Design review of the part built by this model. Coordinates are the model's own, in mm. Face numbers are marked on the shaded views. Round coordinates to 2 decimals unless told otherwise and drop trailing zeros. Order: outer loops, then holes, each group sorted by start corner. A loop starts at its lowest first (then second) coordinate and runs counter-clockwise, first axis right, second up.
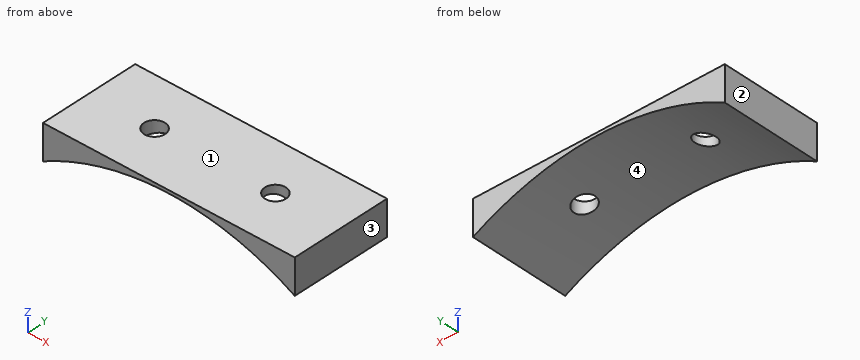
from build123d import *

# Parameters (mm, degrees)
EXTRUDE_1_DEPTH     = 20
SKETCH_2_R          = 2.1
CUT_EXTRUDE_1_DEPTH = 20


with BuildPart() as part:
    # Эскиз1 → Бобышка-Вытянуть1 (new body)
    with BuildSketch(Plane(origin=(0, 0, 0), x_dir=(1, 0, 0), z_dir=(0, 1, 0))):
        with BuildLine():
            Line((-25, -46.165463282), (-25, -53.1))
            Line((-25, -53.1), (25, -53.1))
            Line((25, -53.1), (25, -46.165463282))
            ThreePointArc((25, -46.165463282), (0, -52.5), (-25, -46.165463282))
        make_face()
    extrude(amount=EXTRUDE_1_DEPTH)

    # Эскиз2 → Вырез-Вытянуть1 (cut)
    with BuildSketch(Plane.XY.offset(53.1)):
        with Locations((-12, 10)):
            Circle(SKETCH_2_R)
        with Locations((12, 10)):
            Circle(SKETCH_2_R)
    extrude(amount=-CUT_EXTRUDE_1_DEPTH, mode=Mode.SUBTRACT)


solid = part.part
1) The part is to be moulded in two halves that separate along X. For the marked faces 1, 2, 3 and 4, say which applies: released by +X, released by -X, zero draft, split by the parting line, or undercut.
Results:
face 1: zero draft
face 2: released by -X
face 3: released by +X
face 4: undercut
2) Take a section at B-B on x = 12. Give the boundary of the cut face in (y, z).
Results:
outline: (0, 51.11) - (7.9, 51.11) - (7.9, 53.1) - (0, 53.1) - close; (12.1, 51.11) - (20, 51.11) - (20, 53.1) - (12.1, 53.1) - close
3) Take a section at A-A on y = 10. Give the boundary of the cut face in (x, z), plus the area to 3 significant figures.
Results:
outline: (-25, 46.17) arc R52.5 cw to (-14.1, 50.57) - (-14.1, 53.1) - (-25, 53.1) - close; (-9.9, 51.56) arc R52.5 cw to (9.9, 51.56) - (9.9, 53.1) - (-9.9, 53.1) - close; (14.1, 50.57) arc R52.5 cw to (25, 46.17) - (25, 53.1) - (14.1, 53.1) - close
area: 116 mm2
4) To check wall thickness, follow line 1 along X through (y, z) = (10, 51.45); line 2 along Y through (x, z) = (-12, 52.2); line 3 along X through (y, z) = (8, 47.5). State the ranges of each line that lie inside material, in increasing order.
Results:
line 1: x = -25 to -14.1, 14.1 to 25
line 2: y = 0 to 7.9, 12.1 to 20
line 3: x = -25 to -22.36, 22.36 to 25
5) Clearance check with flat-ended pins moving along their axes: P1, Ø1, axis at x = 15.5, z = 48, coming from the +Y side; P2, Ø2, axis at x = 17, y = 11, coming from the -Z side. State where each tip first meets the part, or that it passes through.
Results:
P1: passes through
P2: stops at z = 49.32
6) Take a section at D-D on z = 52. Give the boundary of the cut face in (x, y), plus the area to 3 significant figures.
Results:
outline: (-25, 0) - (-7.23, 0) - (-7.23, 20) - (-25, 20) - close; (7.23, 0) - (25, 0) - (25, 20) - (7.23, 20) - close; hole circle Ø4.2 at (-12, 10); hole circle Ø4.2 at (12, 10)
area: 683 mm2
7) Take a section at C-C on z = 49.25. Give the boundary of the cut face in (x, y).
Results:
outline: (-25, 0) - (-18.18, 0) - (-18.18, 20) - (-25, 20) - close; (18.18, 0) - (25, 0) - (25, 20) - (18.18, 20) - close
